from build123d import *

# Parameters (mm, degrees)
F0_W     = 105.8307476342
F0_H     = 70.8000324667
F1_DEPTH = 25.4
F2_R     = 18.2213910868
F3_DEPTH = 106.25713
F3_TAPER = 3


# Not quite as in the source:
# - the program builds the solid bodies; features that only make, move or delete a surface that nothing else refers to are left out


with BuildPart() as f1:
    # F0 (on Front) → F1 (new body)
    with BuildSketch(Plane.XZ):
        with Locations((-15.6768169254, 19.381063059)):
            Rectangle(F0_W, F0_H)
    extrude(amount=F1_DEPTH)

    # F2 (on face) → F3 (join)
    with BuildSketch(Plane.XZ.offset(25.4)):
        with Locations((-40.1370152831, 28.4684468061)):
            Circle(F2_R)
    extrude(amount=F3_DEPTH, taper=F3_TAPER)


solid = f1.part
Build history of the part. All positions in model axes, mm. Give positions to 0.01 mm unless a question says otherwise; leave off trailing zeros. Order: outer loops, then holes, each group sorted by start corner. A loop starts at its lowest first (then second) coordinate and runs counter-clockwise, first axis right, second up. Notation, with made-up numbers: M 87,1 L 116,1 A7 ccw 116,10 Z; hole C -4.5,20.5 d8. An arc over 180 degrees is marked long. Put each result on its own line as item: value.
Item 1: Cut at A-A on z = -0.5. Write the cut outline in (x, y), then the cut area to 3 significant figures.
Results are:
outline: M -68.59,-25.4 L 37.24,-25.4 L 37.24,0 L -68.59,0 Z
area: 2,690 mm2
Item 2: Wall check: probe 1 along Y at (x, z) = (19, 19); probe 2 along Z at (x, y) = (-46, -77.5); probe 3 along X at (y, z) = (-99.5, 26.5). Give the ranges that are in metal, low to high.
Results are:
probe 1: -25.4 to 0
probe 2: 14.13 to 42.81
probe 3: -54.34 to -25.93
Item 3: Cut at D-D on y = -105. Write the cut outline in (x, z).
Results are:
outline: C -40.14,28.47 d28.1
Item 4: Cut at C-C on y = -46. Write the cut outline in (x, z), then the cut area to 3 significant figures.
Results are:
outline: C -40.14,28.47 d34.28
area: 923 mm2
Item 5: Cut at B-B on x = -18.5. Write the cut outline in (y, z).
Results are:
outline: M -25.4,-16.02 L 0,-16.02 L 0,54.78 L -25.4,54.78 Z
Item 6: Drop flat-ended pins along their axis: pin 1 Ø1 at (x, z) = (19.5, -4) entering from -Y; pin 2 Ø1.5 at (y, z) = (-28.5, 18) entering from -X; pin 3 Ø8 at (y, z) = (-55.5, 23.5) entering from -X. Give the stop position or say it passes through.
Results are:
pin 1: y = -25.4
pin 2: x = -55.36
pin 3: x = -56.82
